from build123d import *

# Parameters (mm, degrees)
BOSS_EXTRU_1_DEPTH      = 5
ESQUISSE2_R             = 1.5
ENL_V_MAT_EXTRU_1_DEPTH = 6
ESQUISSE3_R             = 1.5
ENL_V_MAT_EXTRU_2_DEPTH = 6
ESQUISSE4_R             = 4
ENL_V_MAT_EXTRU_3_DEPTH = 6


with BuildPart() as part:
    # Esquisse1 → Boss.-Extru.1 (new body)
    with BuildSketch(Plane(origin=(0, 0, 0), x_dir=(1, 0, 0), z_dir=(0, 1, 0))):
        with BuildLine():
            Line((-51.1, -39), (0, -39))
            ThreePointArc((0, -39), (27.577164466, -27.577164466), (39, 0))
            Line((39, 0), (39, 64.082873123))
            Line((39, 64.082873123), (24, 79.082873123))
            Line((24, 79.082873123), (-17.715268603, 79.082873123))
            ThreePointArc((-17.715268603, 79.082873123), (-28.51615758, 26.652464115), (-63.070954357, -14.232410975))
            ThreePointArc((-63.070954357, -14.232410975), (-67.528277829, -27.659845058), (-56.1, -36))
            Line((-56.1, -36), (-51.1, -36))
            Line((-51.1, -36), (-51.1, -39))
        make_face()
    extrude(amount=BOSS_EXTRU_1_DEPTH)

    # Esquisse2 → Enlèv. mat.-Extru.1 (cut, through all)
    with BuildSketch(Plane.XZ):
        with Locations((20.859650045, 20.859650045)):
            Circle(ESQUISSE2_R)
        with Locations((20.859650045, -20.859650045)):
            Circle(ESQUISSE2_R)
        with Locations((-20.859650045, -20.859650045)):
            Circle(ESQUISSE2_R)
        with Locations((-20.859650045, 20.859650045)):
            Circle(ESQUISSE2_R)
        with Locations((17.4, -74.082873123)):
            Circle(ESQUISSE2_R)
        with Locations((17.4, 9.717126877)):
            Circle(ESQUISSE2_R)
    extrude(amount=-ENL_V_MAT_EXTRU_1_DEPTH, mode=Mode.SUBTRACT)

    # Esquisse3 → Enlèv. mat.-Extru.2 (cut, through all)
    with BuildSketch(Plane(origin=(0, 5, 0), x_dir=(1, 0, 0), z_dir=(0, 1, 0))):
        with Locations((17.4, 51.082873123)):
            Circle(ESQUISSE3_R)
        with Locations((-43.1, -9.717126877)):
            Circle(ESQUISSE3_R)
    extrude(amount=-ENL_V_MAT_EXTRU_2_DEPTH, mode=Mode.SUBTRACT)

    # Esquisse4 → Enlèv. mat.-Extru.3 (cut, through all)
    with BuildSketch(Plane(origin=(0, 5, 0), x_dir=(1, 0, 0), z_dir=(0, 1, 0))):
        with Locations((-60.1, -25.917126877)):
            Circle(ESQUISSE4_R)
    extrude(amount=-ENL_V_MAT_EXTRU_3_DEPTH, mode=Mode.SUBTRACT)


solid = part.part
Read the model definition and answer for the solid it produces. Units are mm, in the model's axes. A direction names the side the tool comes from. Coordinates: 2 decimals unless noted, no trailing zeros. Loops run counter-clockwise (first coordinate to the right, second up) from the corner with the lowest first, then second, coordinate; pieces in that order, holes last. Notation, with made-up numbers: (-31, 79) -> (-21, 79) arc R18 ccw to (-21, 112) -> close; hole circle Ø9 at (40.25, 56.25). An arc over 180 degrees is marked (long way). Answer in a Markdown table with one row per item.
Item 1: Straight lines are drawn through the part: line 1 along X through (y, z) = (1.6, 25); line 2 along Z through (x, y) = (1.5, 0.4); line 3 along X through (y, z) = (4.6, -50.5). For each, find the intervals that lie inside material, in ascending order. Write a range as [from, to].
Returned:
| item | result |
|---|---|
| line 1 | x = [-68.06, -63.99], [-56.21, 29.93] |
| line 2 | z = [-79.08, 38.97] |
| line 3 | x = [-20.19, 16.02], [18.78, 39] |
Item 2: A cutting plane is placed at B-B on y = 4.25. Give the number of separate pieces and of enclosed holes in the cut face, plus the area to 3 significant figures.
Returned:
| item | result |
|---|---|
| separate pieces | 1 |
| enclosed holes | 9 |
| area | 8,490 mm^2 |
Item 3: A cutting plane is placed at A-A on x = -60.1. Determine the outline of the cut face in (y, z).
Returned:
| item | result |
|---|---|
| outline | (0, 12.03) -> (5, 12.03) -> (5, 21.92) -> (0, 21.92) -> close; (0, 29.92) -> (5, 29.92) -> (5, 35.31) -> (0, 35.31) -> close |
Item 4: A cutting plane is placed at C-C on x = -43.1. Determine the outline of the cut face in (y, z), plus the area to 3 significant figures.
Returned:
| item | result |
|---|---|
| outline | (0, -4.2) -> (5, -4.2) -> (5, 8.22) -> (0, 8.22) -> close; (0, 11.22) -> (5, 11.22) -> (5, 39) -> (0, 39) -> close |
| area | 201 mm^2 |
Item 5: Each of these flat-tipped pins is pushed along its axis until it touches: P1, Ø1.5, axis at y = 1.5, z = 12, coming from the +X side; P2, Ø1, axis at y = 1, z = 25, coming from the -X side; P3, Ø1.8, axis at x = -43.1, z = 9.72, coming from the -Y side; P4, Ø1, axis at y = 3, z = -16.5, coming from the -X side. Where does it stop, or does it pass through?
Returned:
| item | result |
|---|---|
| P1 | stops at x = 37.34 |
| P2 | stops at x = -68.09 |
| P3 | passes through |
| P4 | stops at x = -34.46 |
Item 6: A cutting plane is placed at D-D on z = 16. Determine the outline of the cut face in (x, y).
Returned:
| item | result |
|---|---|
| outline | (-65.04, 0) -> (35.57, 0) -> (35.57, 5) -> (-65.04, 5) -> close |
Item 7: For a pull along X with two mould halves and no side action, classify faces 3 (the cylindrical face through (27.27, 2.46, 27.88)), 4 (the flat face through (-3, 0, -8)), 5 (the cylindrical face through (18.21, 2.46, -72.82)) as released by +X, released by -X, zero draft, split by the parting line, or undercut.
Returned:
| item | result |
|---|---|
| face 3 | released by +X |
| face 4 | zero draft |
| face 5 | undercut |
Item 8: For faces 1 (the cylindrical face through (-56.285, 2.535, 24.716)), 2 (the flat face through (-51.1, 2, 37)), determine the directions among +Z, -Z, +X, -X, +Y, -Y from which every point of the face is accessible in a straight line to the end or side of a thin tool.
Returned:
| item | result |
|---|---|
| face 1 | +Y, -Y |
| face 2 | +Z, -X, +Y, -Y |
